Study the drawing (mm; zero at the part's minimum x, y, z) and answer. Coordinates: 2 decimals unless noted, no trailing zeros. Order: outer loops, then holes, each group sorted by start corner. A loop starts at its lowest first (then second) coordinate and runs counter-clockwise, first axis right, second up.
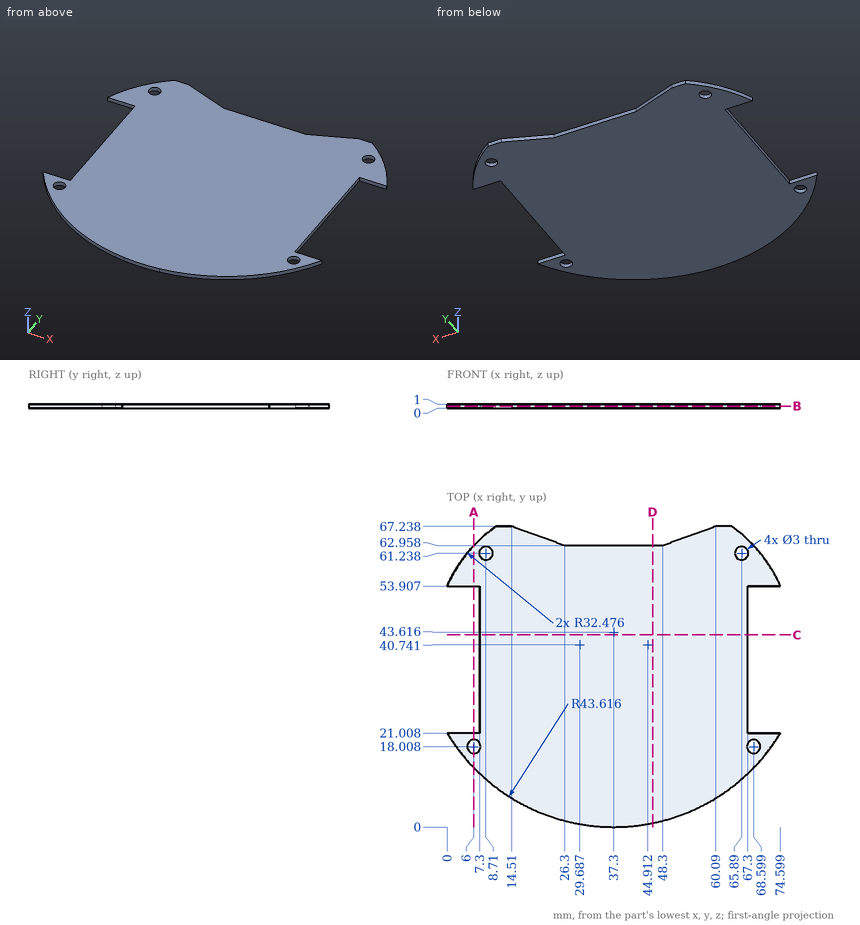
1) A cutting plane is placed at B-B, the plane z = 0.55. Determine the outline of the cut face in (x, y) (1 decimal).
A:
outline: (0, 21) arc R43.6 ccw to (74.6, 21) - (67.3, 21) - (67.3, 53.9) - (74.6, 53.9) arc R32.5 ccw to (63.7, 67.2) - (60.1, 67.2) - (48.3, 63) - (26.3, 63) - (14.5, 67.2) - (10.9, 67.2) arc R32.5 ccw to (0, 53.9) - (7.3, 53.9) - (7.3, 21) - close; hole circle Ø3 at (6, 18); hole circle Ø3 at (8.7, 61.2); hole circle Ø3 at (65.9, 61.2); hole circle Ø3 at (68.6, 18)
2) Straight lines are drawn through the part: line 1 (Y direction, x = 6, z = 0.4) (1 decimal); line 2 (Y direction, x = 5.5, z = 0.1) (1 decimal); line 3 (X direction, y = 29.5, z = 0.75). For each, find the intervals that lie inside material, in ascending order.
A:
line 1: y = 13.2 to 16.5, 19.5 to 21, 53.9 to 63
line 2: y = 13.8 to 16.6, 19.4 to 21, 53.9 to 62.4
line 3: x = 7.3 to 67.3
3) A cutting plane is placed at C-C, the plane y = 43. Determine the outline of the cut face in (x, z).
A:
outline: (7.3, 0) - (67.3, 0) - (67.3, 1) - (7.3, 1) - close
4) A cutting plane is placed at D-D, the plane x = 46. Determine the outline of the cut face in (y, z).
A:
outline: (0.88, 0) - (62.96, 0) - (62.96, 1) - (0.88, 1) - close
5) A cutting plane is placed at A-A, the plane x = 6. Determine the outline of the cut face in (y, z).
A:
outline: (13.24, 0) - (16.51, 0) - (16.51, 1) - (13.24, 1) - close; (19.51, 0) - (21.01, 0) - (21.01, 1) - (19.51, 1) - close; (53.91, 0) - (62.96, 0) - (62.96, 1) - (53.91, 1) - close
6) Flat-ended cylindrical pins translate along their axes: pin 1 Ø0.5 at (y, z) = (41, 0.5) entering from -X; pin 2 Ø0.5 at (x, z) = (72, 0.5) entering from -Y (1 decimal); pin 3 Ø0.5 at (x, z) = (3.5, 0.5) entering from +Y (1 decimal). Find the tip coordinate at first contact, or state that the pin passes through.
A:
pin 1: stops at x = 7.3
pin 2: stops at y = 16.9
pin 3: stops at y = 60.3
